Print and shaded views of the part. All mm, measured from the part's lowest x, y and z. A direction names the side the tool comes from. Give positions to 0.01 mm unless a question says otherwise; leave off trailing zeros. Loops run counter-clockwise (first coordinate to the right, second up) from the corner with the lowest first, then second, coordinate; pieces in that order, holes last. Notation, with made-up numbers: (51.25, -38) - (70.25, -38) arc R16 cw to (70.25, -9) - close; hole circle Ø10 at (-19, 45). An arc over 180 degrees is marked (long way). Return JSON: item names as keys, results as strings.
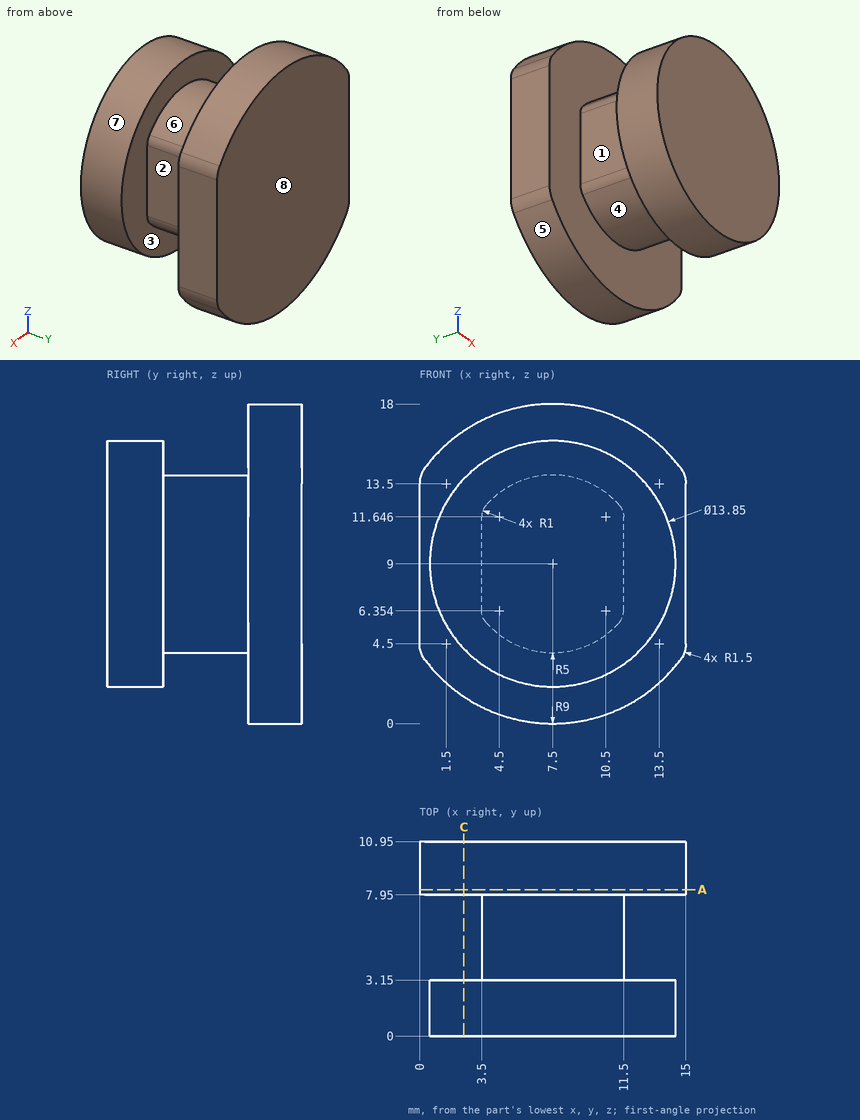
1. Drill centre lines: probe 1 along Y at (x, z) = (8, 15.5); probe 2 along Z at (x, y) = (7.5, 6.25); probe 3 along Y at (x, z) = (3.25, 16). Where is each one in solid material? Low to high.
Values follow:
{"probe 1": "y = 0 to 3.15, 7.95 to 10.95", "probe 2": "z = 4 to 14", "probe 3": "y = 7.95 to 10.95"}
2. Drop flat-ended pins along their axis: P1, Ø1.5, axis at x = 7.5, y = 1, coming from the -Z side (3 decimals); P2, Ø4, axis at x = 11.5, y = 6.5, coming from the +Z side; P3, Ø1.4, axis at y = 5.5, z = 10, coming from the -X side. Give the stop position or say it passes through.
Values follow:
{"P1": "stops at z = 2.075", "P2": "stops at z = 17.61", "P3": "stops at x = 3.5"}
3. Which spindle directions (+Z, -Z, +X, -X, +Y, -Y) get a long thin tool onto all of the face, cutting with end or side? Do the marked faces 1, 2, 3, 4 and 5. Say none if no direction does.
Values follow:
{"face 1": "+Z, -Z, -X", "face 2": "+Z, -Z, +X", "face 3": "none", "face 4": "-Z", "face 5": "-Z, +Y, -Y"}
4. Pull direction Y, two halves, no side cores. Call the marked faces 6, 7 and 8: +Y half, -Y half, draft (parallel to the pull), parting line (faces both ways), or undercut.
Values follow:
{"face 6": "undercut", "face 7": "draft", "face 8": "+Y half"}
5. Cut at C-C, the plane x = 2.5. Write the cut outline in (y, z), plus the area to 3 significant figures.
Values follow:
{"outline": "(0, 4.21) - (3.15, 4.21) - (3.15, 13.79) - (0, 13.79) - close; (7.95, 1.52) - (10.95, 1.52) - (10.95, 16.48) - (7.95, 16.48) - close", "area": "75.1 mm²"}
6. Cut at A-A, the plane y = 8.25. Write the cut outline in (x, z), plus the area to 3 significant figures.
Values follow:
{"outline": "(0, 4.5) arc R1.5 ccw to (0.3, 3.6) arc R9 ccw to (14.7, 3.6) arc R1.5 ccw to (15, 4.5) - (15, 13.5) arc R1.5 ccw to (14.7, 14.4) arc R9 ccw to (0.3, 14.4) arc R1.5 ccw to (0, 13.5) - close", "area": "234 mm²"}
